Autodesk Inventor part; units mm, degrees
ref_plane "YZ Plane" through (0, 0, 0) normal (1, 0, 0) x (0, 1, 0)
ref_plane "XZ Plane" through (0, 0, 0) normal (0, 1, 0) x (-1, 0, 0)
ref_plane "XY Plane" through (0, 0, 0) normal (0, 0, 1) x (1, 0, 0)
sketch "Эскиз1" plane through (0, 0, 0) normal (0, 1, 0) x (-1, 0, 0)
  line L0 (9.3708, 3) -> (9.3708, -3)
  line L1 (9.3708, -3) -> (9.3708, -4.5)
  arc A0 (8.3708, -5.5) -> (9.3708, -4.5) centre (8.3708, -4.5) ccw
  line L2 (8.3708, -5.5) -> (-0.6292, -5.5)
  arc A1 (-1.6292, -4.5) -> (-0.6292, -5.5) centre (-0.6292, -4.5) ccw
  line L3 (-1.6292, -4.5) -> (-1.6292, -3)
  arc A2 (-1.6292, -3) -> (-2.1292, -2.5) centre (-2.1292, -3) ccw
  line L4 (-3.1292, -2.5) -> (-2.1292, -2.5)
  arc A3 (-3.6292, -2) -> (-3.1292, -2.5) centre (-3.1292, -2) ccw
  line L5 (-3.6292, 2) -> (-3.6292, -2)
  arc A4 (-3.1292, 2.5) -> (-3.6292, 2) centre (-3.1292, 2) ccw
  line L6 (-2.1292, 2.5) -> (-3.1292, 2.5)
  arc A5 (-2.1292, 2.5) -> (-1.6292, 3) centre (-2.1292, 3) ccw
  line L7 (-1.6292, 3) -> (-1.6292, 4.5)
  arc A6 (-0.6292, 5.5) -> (-1.6292, 4.5) centre (-0.6292, 4.5) ccw
  line L8 (-0.6292, 5.5) -> (8.3708, 5.5)
  arc A7 (9.3708, 4.5) -> (8.3708, 5.5) centre (8.3708, 4.5) ccw
  line L9 (9.3708, 4.5) -> (9.3708, 3)
  arc A8 (6.8708, 1.5) -> (5.3708, 3) centre (5.3708, 1.5) ccw
  line L10 (2.3708, 3) -> (5.3708, 3)
  arc A9 (2.3708, 3) -> (0.8708, 1.5) centre (2.3708, 1.5) ccw
  line L11 (0.8708, -1.5) -> (0.8708, 1.5)
  arc A10 (0.8708, -1.5) -> (2.3708, -3) centre (2.3708, -1.5) ccw
  line L12 (5.3708, -3) -> (2.3708, -3)
  arc A11 (5.3708, -3) -> (6.8708, -1.5) centre (5.3708, -1.5) ccw
  line L13 (6.8708, 1.5) -> (6.8708, -1.5)
  arc A12 (9.8708, -2.5) -> (9.3708, -3) centre (9.8708, -3) ccw
  line L14 (9.3708, 3) -> (9.3708, -3)
  arc A13 (9.3708, 3) -> (9.8708, 2.5) centre (9.8708, 3) ccw
  line L15 (10.8708, 2.5) -> (9.8708, 2.5)
  arc A14 (11.3708, 2) -> (10.8708, 2.5) centre (10.8708, 2) ccw
  line L16 (11.3708, -2) -> (11.3708, 2)
  arc A15 (10.8708, -2.5) -> (11.3708, -2) centre (10.8708, -2) ccw
  line L17 (9.8708, -2.5) -> (10.8708, -2.5)
  line L18 (9.0708, 3) -> (9.0708, 4.5)
  arc A16 (9.0708, 4.5) -> (8.3708, 5.2) centre (8.3708, 4.5) ccw
  line L19 (8.3708, 5.2) -> (-0.6292, 5.2)
  arc A17 (-0.6292, 5.2) -> (-1.3292, 4.5) centre (-0.6292, 4.5) ccw
  line L20 (-1.3292, 4.5) -> (-1.3292, 3)
  arc A18 (-2.1292, 2.2) -> (-1.3292, 3) centre (-2.1292, 3) ccw
  line L21 (-2.1292, 2.2) -> (-3.1292, 2.2)
  arc A19 (-3.1292, 2.2) -> (-3.3292, 2) centre (-3.1292, 2) ccw
  line L22 (-3.3292, 2) -> (-3.3292, -2)
  arc A20 (-3.3292, -2) -> (-3.1292, -2.2) centre (-3.1292, -2) ccw
  line L23 (-3.1292, -2.2) -> (-2.1292, -2.2)
  arc A21 (-1.3292, -3) -> (-2.1292, -2.2) centre (-2.1292, -3) ccw
  line L24 (-1.3292, -3) -> (-1.3292, -4.5)
  arc A22 (-1.3292, -4.5) -> (-0.6292, -5.2) centre (-0.6292, -4.5) ccw
  line L25 (-0.6292, -5.2) -> (8.3708, -5.2)
  arc A23 (8.3708, -5.2) -> (9.0708, -4.5) centre (8.3708, -4.5) ccw
  line L26 (9.0708, -4.5) -> (9.0708, -3)
  arc A24 (9.0708, 3) -> (9.8708, 2.2) centre (9.8708, 3) ccw
  line L27 (9.8708, 2.2) -> (10.8708, 2.2)
  arc A25 (11.0708, 2) -> (10.8708, 2.2) centre (10.8708, 2) ccw
  line L28 (11.0708, 2) -> (11.0708, -2)
  arc A26 (10.8708, -2.2) -> (11.0708, -2) centre (10.8708, -2) ccw
  line L29 (10.8708, -2.2) -> (9.8708, -2.2)
  arc A27 (9.8708, -2.2) -> (9.0708, -3) centre (9.8708, -3) ccw
  point P0 (0, 0)
  dimension "d0" = 0.3
  dimension "d1" = 0.3
extrude "Выдавливание1" add sketch "Эскиз1" along normal blind 1 contours A24 L27 A25 L28 A26 L29 A27 L0 | L0 A27 L26 A23 L25 A22 L24 A21 L23 A20 L22 A19 L21 A18 L20 A17 L19 A16 L18 A24 | L13 A11 L12 A10 L11 A9 L10 A8
sketch "Эскиз2" plane through (0, 0, 0) normal (0, -1, 0) x (1, 0, 0)
  arc A0 (-8.3708, 5.2) -> (-9.0708, 4.5) centre (-8.3708, 4.5) ccw
  line L0 (-9.0708, 3) -> (-9.0708, 4.5)
  arc A1 (-9.8708, 2.2) -> (-9.0708, 3) centre (-9.8708, 3) ccw
  line L1 (-10.8708, 2.2) -> (-9.8708, 2.2)
  arc A2 (-10.8708, 2.2) -> (-11.0708, 2) centre (-10.8708, 2) ccw
  line L2 (-11.0708, -2) -> (-11.0708, 2)
  arc A3 (-11.0708, -2) -> (-10.8708, -2.2) centre (-10.8708, -2) ccw
  line L3 (-9.8708, -2.2) -> (-10.8708, -2.2)
  arc A4 (-9.0708, -3) -> (-9.8708, -2.2) centre (-9.8708, -3) ccw
  line L4 (-9.0708, -4.5) -> (-9.0708, -3)
  arc A5 (-9.0708, -4.5) -> (-8.3708, -5.2) centre (-8.3708, -4.5) ccw
  line L5 (0.6292, -5.2) -> (-8.3708, -5.2)
  arc A6 (0.6292, -5.2) -> (1.3292, -4.5) centre (0.6292, -4.5) ccw
  line L6 (1.3292, -3) -> (1.3292, -4.5)
  arc A7 (2.1292, -2.2) -> (1.3292, -3) centre (2.1292, -3) ccw
  line L7 (3.1292, -2.2) -> (2.1292, -2.2)
  arc A8 (3.1292, -2.2) -> (3.3292, -2) centre (3.1292, -2) ccw
  line L8 (3.3292, 2) -> (3.3292, -2)
  arc A9 (3.3292, 2) -> (3.1292, 2.2) centre (3.1292, 2) ccw
  line L9 (2.1292, 2.2) -> (3.1292, 2.2)
  arc A10 (1.3292, 3) -> (2.1292, 2.2) centre (2.1292, 3) ccw
  line L10 (1.3292, 4.5) -> (1.3292, 3)
  arc A11 (1.3292, 4.5) -> (0.6292, 5.2) centre (0.6292, 4.5) ccw
  line L11 (-8.3708, 5.2) -> (0.6292, 5.2)
  arc A12 (-9.8708, 2.2) -> (-9.0708, 3) centre (-9.8708, 3) ccw
  line L12 (-9.0708, -3) -> (-9.0708, 3)
  line L13 (1.3292, 3) -> (1.3292, -3)
  point P0 (0, 0)
extrude "Выдавливание2" add sketch "Эскиз2" along normal blind 4 contours L11 A11 L10 L13 L6 A6 L5 A5 L4 L12 L0 A0
sketch "Эскиз3" plane through (-9.0708, 0, -3) normal (-1, 0, 0) x (0, 0, 1)
  line L0 (0, 0) -> (0, 1)
  line L1 (-1.5, 1) -> (0, 1)
  line L2 (-1.5, -4) -> (-1.5, 1)
  line L3 (7.5, -4) -> (-1.5, -4)
  line L4 (7.5, 1) -> (7.5, -4)
  line L5 (6, 1) -> (7.5, 1)
  line L6 (6, 0) -> (6, 1)
  line L7 (0, 0) -> (6, 0)
  line L8 (7.5, 1) -> (8.2, 1)
  line L9 (7.5, 1) -> (7.5, -4)
  line L10 (-1.5, -4) -> (-1.5, 1)
  line L11 (-2.2, 1) -> (-1.5, 1)
  line L12 (-2.2, -4) -> (-2.2, 1)
  line L13 (-1.5, -4) -> (-2.2, -4)
  line L14 (8.2, 1) -> (7.5, 1)
  line L15 (8.2, -1.5) -> (4.6296, -4)
  line L16 (7.5, -4) -> (-1.5, -4)
  line L17 (-1.5, 1) -> (-2.2, 1)
  line L18 (-2.2, 1) -> (-2.2, -1.5)
  line L19 (-2.2, -4) -> (-2.2, 1)
  line L20 (-2.2, -1.5) -> (1.3704, -4)
  line L21 (7.5, 1) -> (7.5, -4)
  line L22 (8.2, -4) -> (8.2, 1)
  line L23 (7.5, -4) -> (8.2, -4)
  line L24 (8.2, 1) -> (8.2, -1.5)
  point P0 (3, 0)
  point P1 (-2.2, -1.5)
  dimension "d8" = 2.5
  dimension "d9" = 35
  dimension "d10" = 35
  dimension "d14" = 2.5
extrude "Выдавливание3" cut sketch "Эскиз3" against normal blind 15 contours L20 L3 L2 | L2 L13 L12 L20 | L15 L22 L23 L4 | L4 L3 L15
fillet "Сопряжение2" radius 1 2 edges at (-3.8708, -4, -1.6296) (-3.8708, -4, 1.6296)
fillet "Сопряжение3" radius 0.5 8 edges at (-9.0708, -2.9046, 3.194) (-8.8657, -1.6436, 4.995) (-3.8708, -1.5, 5.2) (1.1242, -1.6436, 4.995) (1.3292, -2.9046, 3.194) (1.1242, -1.6436, -4.995) (-3.8708, -1.5, -5.2) (-8.8657, -1.6436, -4.995)
properties part number "pinatel"
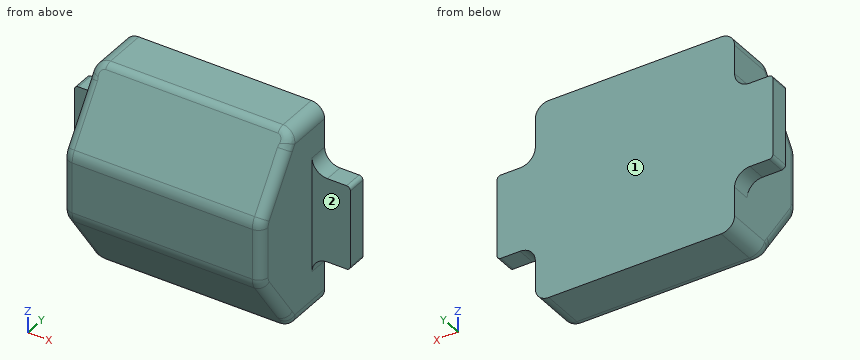
CAD build for the part. Positions are in the model's coordinates, mm. Face numbers are marked on the shaded views. A direction names the side the tool comes from. Give positions to 0.01 mm unless a question says otherwise; leave off trailing zeros. Write each loop counter-clockwise with the first axis right and the second up, starting at its lowest first coordinate (ties: lowest second). Pieces come first, ordered by that corner, then holes. Notation, with made-up numbers: M -21,10 L 0,10 A28 ccw 0,41 Z; hole C -34,37.25 d7. An arc over 180 degrees is marked long. Return JSON: item names as keys, results as strings. Group by question number.
(1) Flat gauge pins, fed straight in: pin 1 Ø3 at (x, z) = (-9.5, -2.5) entering from -Y; pin 2 Ø0.8 at (x, y) = (2.5, 0.5) entering from +Z; pin 3 Ø1.6 at (x, z) = (-10.5, 0.5) entering from -Y; pin 4 Ø2.5 at (y, z) = (-2, 1) entering from -X. Where does each tip first touch, or does it go through?
(2) Band-saw the part on A-A (z = -1). Give the cut face in (x, y).
(3) Drill centre lines: L1, parallel to X at y = -0.9, z = -1.5; L2, parallel to Y at x = -10.5, z = -2; L3, parallel to Z at x = -10, y = 0.5. Where is each one in solid material? Low to high. Write a range as [from, to].
(4) 3-axis set-ups, long thin cutter, end or side, ignore diameter. For the marked faces 1 and 2: which of +Z, -Z, +X, -X, +Y, -Y reach the whole face in a straight line?
(5) Band-saw the part on C-C (x = -3.25). Give the cut face in (y, z).
(6) Band-saw the part on B-B (y = -1.05). Give the cut face in (x, z).
Entries:
{
 "1": {"pin 1": "stops at y = -4", "pin 2": "stops at z = 2.2", "pin 3": "stops at y = 0", "pin 4": "stops at x = -9.07"},
 "2": {"outline": "M -11.07,0 L -9.07,0 L -9.07,-3.5 A0.5 ccw -8.57,-4 L 0.83,-4 A0.5 ccw 1.33,-3.5 L 1.33,0 L 3.33,0 L 3.33,1 L -11.07,1 Z"},
 "3": {"L1": "x = [-9.07, 1.33]", "L2": "y = [0, 1]", "L3": "z = [-2.2, 2.2]"},
 "4": {"face 1": "+Z, -Z, +X, -X, +Y", "face 2": "+Z, -Z, +X, -Y"},
 "5": {"outline": "M -4,-1.31 A1 ccw -3.82,-1.89 L -1.65,-4.99 A0.5 ccw -1.24,-5.2 L 1,-5.2 L 1,5.2 L -1.24,5.2 A0.5 ccw -1.65,4.99 L -3.82,1.89 A1 ccw -4,1.31 Z"},
 "6": {"outline": "M -9.07,-4.5 A0.7 ccw -8.37,-5.2 L 0.63,-5.2 A0.7 ccw 1.33,-4.5 L 1.33,4.5 A0.7 ccw 0.63,5.2 L -8.37,5.2 A0.7 ccw -9.07,4.5 Z"}
}
